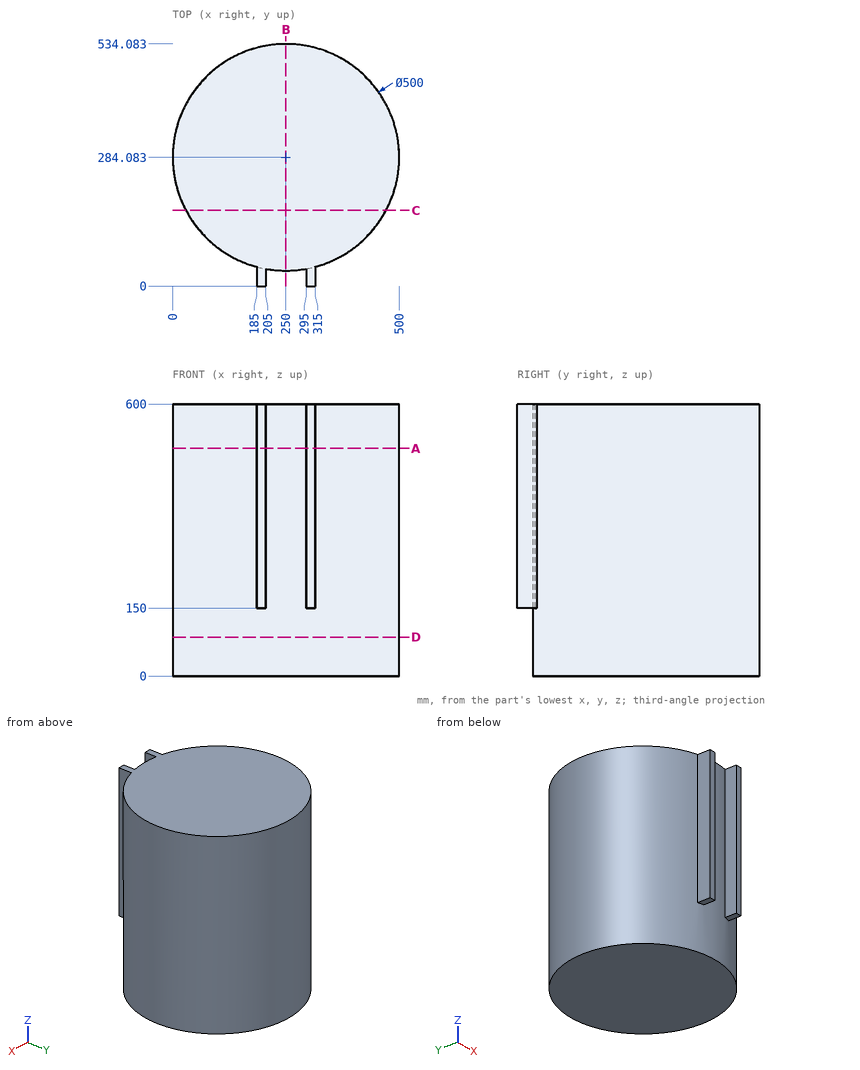
Source: three-view drawing plus pictorial views. Frame: mm from the lowest corner of the part. Round coordinates to 2 decimals unless told otherwise and drop trailing zeros. Write each loop counter-clockwise with the first axis right and the second up, starting at its lowest first coordinate (ties: lowest second). Pieces come first, ordered by that corner, then holes. Notation, with made-up numbers: M 55,32.25 L 70,32.25 A28 cw 70,59.25 Z; hole C 63,1.5 d8. An arc over 180 degrees is marked long. One line per item, written item: value. Start each with the question number.
Item 1: Section query D-D (z = 86). Return the cut outline in (x, y).
Item 2: Ray query, L1, parallel to X at y = 22.5, z = 302.5; L2, parallel to X at y = 281.5, z = 238.5; L3, parallel to Y at x = 253.5, z = 501. Return the intervals inside material, ascending. Write a range as from..to.
Item 3: Section query C-C (y = 167). Return the cut outline in (x, z).
Item 4: Section query B-B (x = 250). Return the cut outline in (y, z), plus the area to 3 significant figures.
Item 5: Pin query (flat end, axial travel): pin 1 (13 mm diameter, centred on y = 28, z = 347.5, fed in from +X); pin 2 (2 mm diameter, centred on y = 466.5, z = 429, fed in from +X); pin 3 (5 mm diameter, centred on x = 135, z = 306, fed in from -Y) (1 decimal). Return the tip coordinate at first contact, or that it passes through.
Item 6: Section query A-A (z = 502). Return the cut outline in (x, y), plus the area to 3 significant figures.
Result set:
1. outline: C 250,284.08 d500
2. L1: x = 185..205, 295..315
2. L2: x = 0.01..499.99
2. L3: y = 34.11..534.06
3. outline: M 29.11,0 L 470.89,0 L 470.89,600 L 29.11,600 Z
4. outline: M 34.08,0 L 534.08,0 L 534.08,600 L 34.08,600 Z
4. area: 300,000 mm²
5. pin 1: stops at x = 315
5. pin 2: stops at x = 422.01
5. pin 3: stops at y = 60.8
6. outline: M 185,0 L 205,0 L 205,38.17 A250 ccw 295,38.17 L 295,0 L 315,0 L 315,42.68 A250 ccw long 185,42.68 Z
6. area: 198,000 mm²
